Answer from the drawing. Dimensions are ordinates in mm from the lowest x, y and z of the part. A direction names the side the tool comes from. Coordinates: 2 decimals unless noted, no trailing zeros. Order: outer loops, then holes, each group sorted by start corner. A loop starts at its lowest first (then second) coordinate and runs counter-clockwise, first axis right, second up. Notation, with made-up numbers: (7.5, -13) - (22.5, -13) arc R22 ccw to (22.5, 13) - close; hole circle Ø1 at (24, 31). An arc over 180 degrees is marked (long way). One line per item, written item: value. Start each with the question number.
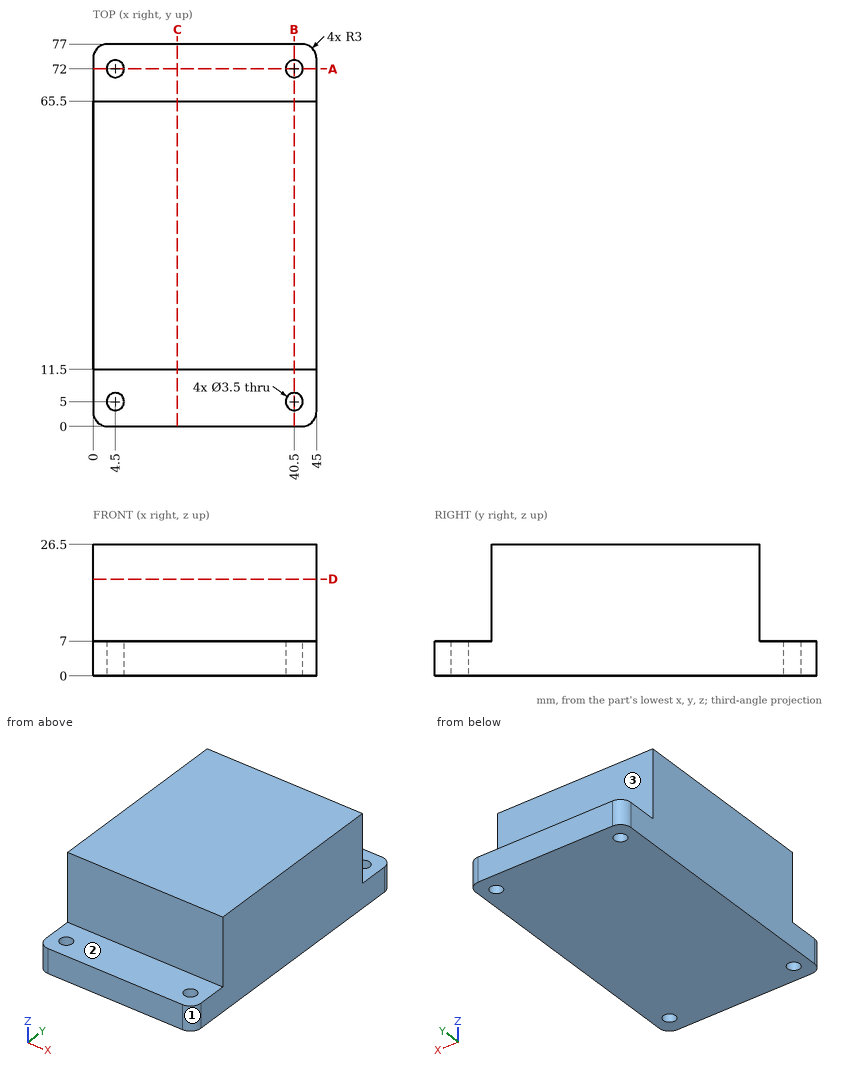
(1) For the marked faces 1, 2 and 3, determine the directions among +Z, -Z, +X, -X, +Y, -Y from which every point of the face is accessible in a straight line to the end or side of a thin tool.
(2) The part is cut by section C-C on x = 17. Determine the outline of the cut face in (y, z), plus the area to 3 significant figures.
(3) Flat-ended cylindrical pins translate along their axes: pin 1 Ø10 at (x, z) = (15, 21) entering from +Y; pin 2 Ø3.5 at (x, y) = (33.5, 4.5) entering from +Z; pin 3 Ø6 at (x, z) = (18, 17) entering from -Y. Find the tip coordinate at first contact, or state that the pin passes through.
(4) The part is cut by section D-D on z = 19.5. Determine the outline of the cut face in (x, y), plus the area to 3 significant figures.
(5) The part is cut by section A-A on y = 72. Determine the outline of the cut face in (x, z).
(6) Consider probe 1 along Y at (x, z) = (4.5, 1.5); probe 2 along X at (y, z) = (72, 3); probe 3 along Z at (x, y) = (38.5, 4). Determine where each line is inside the solid, lowest interval first.
(7) The part is cut by section B-B on x = 40.5. Determine the outline of the cut face in (y, z).
Completed:
1. face 1: +Z, -Z, +X, -Y
1. face 2: +Z, +X, -X, -Y
1. face 3: +Z, +X, -X, +Y
2. outline: (0, 0) - (77, 0) - (77, 7) - (65.5, 7) - (65.5, 26.5) - (11.5, 26.5) - (11.5, 7) - (0, 7) - close
2. area: 1,590 mm2
3. pin 1: stops at y = 65.5
3. pin 2: stops at z = 7
3. pin 3: stops at y = 11.5
4. outline: (0, 11.5) - (45, 11.5) - (45, 65.5) - (0, 65.5) - close
4. area: 2,430 mm2
5. outline: (0, 0) - (2.75, 0) - (2.75, 7) - (0, 7) - close; (6.25, 0) - (38.75, 0) - (38.75, 7) - (6.25, 7) - close; (42.25, 0) - (45, 0) - (45, 7) - (42.25, 7) - close
6. probe 1: y = 0 to 3.25, 6.75 to 70.25, 73.75 to 77
6. probe 2: x = 0 to 2.75, 6.25 to 38.75, 42.25 to 45
6. probe 3: z = 0 to 7
7. outline: (0, 0) - (3.25, 0) - (3.25, 7) - (0, 7) - close; (6.75, 0) - (70.25, 0) - (70.25, 7) - (65.5, 7) - (65.5, 26.5) - (11.5, 26.5) - (11.5, 7) - (6.75, 7) - close; (73.75, 0) - (77, 0) - (77, 7) - (73.75, 7) - close
